Autodesk Inventor part; units mm, degrees
ref_plane "YZ Plane" through (0, 0, 0) normal (1, 0, 0) x (0, 1, 0)
ref_plane "XZ Plane" through (0, 0, 0) normal (0, 1, 0) x (-1, 0, 0)
ref_plane "XY Plane" through (0, 0, 0) normal (0, 0, 1) x (1, 0, 0)
sketch "Sketch1" plane through (0, 0, 0) normal (0, 1, 0) x (-1, 0, 0)
  line L0 (-81.5, 81.5) -> (81.5, -81.5) construction
  line L1 (-81.5, -81.5) -> (81.5, 81.5) construction
  line L2 (-66.3, 66.3) -> (66.3, -66.3) construction
  line L3 (-66.3, -66.3) -> (66.3, 66.3) construction
  line L4 (-81.9, 81.9) -> (-81.9, -81.9)
  line L5 (-81.9, -81.9) -> (81.9, -81.9)
  line L6 (81.9, -81.9) -> (81.9, 81.9)
  line L7 (81.9, 81.9) -> (-81.9, 81.9)
  line L8 (-66.1, 66.1) -> (-66.1, -66.1)
  line L9 (-66.1, -66.1) -> (66.1, -66.1)
  line L10 (66.1, -66.1) -> (66.1, 66.1)
  line L11 (66.1, 66.1) -> (-66.1, 66.1)
  line L12 (-66.1, 66.1) -> (66.1, -66.1) construction
  line L13 (-66.1, -66.1) -> (66.1, 66.1) construction
  line L14 (66.1, 51.9579) -> (17.2261, 3.084)
  line L15 (51.9579, 66.1) -> (3.084, 17.2261)
  line L16 (66.1, -51.9579) -> (14.1421, 0) construction
  line L17 (50.106, -64.2481) -> (3.084, -17.2261)
  arc A0 (-17.2261, -3.084) -> (-3.084, -17.2261) centre (0, 0) ccw
  arc A1 (-17.2261, 3.084) -> (-17.2261, -3.084) centre (0, 0) ccw
  line L18 (-14.1421, 0) -> (-17.2261, -3.084) construction
  line L19 (-3.084, 17.2261) -> (-51.9579, 66.1)
  line L20 (3.084, 17.2261) -> (0, 14.1421) construction
  line L21 (0, 14.1421) -> (-14.1421, 0) construction
  line L22 (14.1421, 0) -> (-3.084, 17.2261) construction
  arc A2 (17.2261, 3.084) -> (-17.2261, 3.084) centre (0, 0) ccw
  arc A3 (17.2261, -3.084) -> (17.2261, 3.084) centre (0, 0) ccw
  arc A4 (-3.084, -17.2261) -> (17.2261, -3.084) centre (0, 0) ccw
  line L23 (3.084, -17.2261) -> (0, -14.1421) construction
  line L24 (0, -14.1421) -> (-14.1421, 0) construction
  line L25 (17.2261, 3.084) -> (-3.084, -17.2261) construction
  line L26 (-3.084, -17.2261) -> (-51.9579, -66.1)
  line L27 (-17.2261, -3.084) -> (-66.1, -51.9579)
  line L28 (-17.2261, 3.084) -> (-64.2481, 50.106)
  line L29 (-14.1421, 0) -> (-17.2261, 3.084) construction
  line L30 (17.2261, -3.084) -> (66.1, -51.9579)
  line L31 (50.106, -64.2481) -> (51.9579, -66.1)
  line L32 (-64.2481, 50.106) -> (-66.1, 51.9579)
  line L33 (46.2, 46.2) -> (-46.2, 46.2) construction
  line L34 (-46.2, 46.2) -> (-46.2, -46.2) construction
  line L35 (-46.2, -46.2) -> (46.2, -46.2) construction
  line L36 (46.2, -46.2) -> (46.2, 46.2) construction
  line L37 (46.2, 46.2) -> (-46.2, -46.2) construction
  line L38 (-46.2, 46.2) -> (46.2, -46.2) construction
  circle A5 centre (46.2, -46.2) radius 1
  circle A6 centre (-46.2, -46.2) radius 1
  circle A7 centre (-46.2, 46.2) radius 1
  circle A8 centre (46.2, 46.2) radius 1
  line L39 (51.9579, 66.1) -> (66.1, 51.9579)
  line L40 (66.1, -51.9579) -> (51.9579, -66.1)
  line L41 (-51.9579, -66.1) -> (-66.1, -51.9579)
  line L42 (-66.1, 51.9579) -> (-51.9579, 66.1)
  line L43 (-74, 74) -> (-74, -74)
  line L44 (-74, -74) -> (74, -74)
  line L45 (74, -74) -> (74, 74)
  line L46 (74, 74) -> (-74, 74)
  line L47 (-74, 74) -> (74, -74) construction
  line L48 (-74, -74) -> (74, 74) construction
  dimension "d0" = 163
  dimension "d1" = 163
  dimension "d2" = 132.6
  dimension "d3" = 132.6
  dimension "d5" = 163.8
  dimension "d6" = 163.8
  dimension "d7" = 132.2
  dimension "d8" = 132.2
  dimension "d9" = 20
  dimension "d10" = 20
  dimension "d11" = 35
  dimension "d12" = 92.4
  dimension "d13" = 92.4
  dimension "d14" = 2
  dimension "d15" = 2
  dimension "d16" = 2
  dimension "d17" = 2
  dimension "d28" = 148
  dimension "d29" = 148
extrude "Extrusion1" add sketch "Sketch1" along normal blind 5 contours L7 L6 L5 L4 | L46 L45 L44 L43
extrude "Extrusion2" add sketch "Sketch1" along normal blind 5 contours L11 L42 L8 | L41 L9 L8 | L11 L10 L39 | L40 L10 L9
extrude "Extrusion4" cut sketch "Sketch1" against normal blind 10 contours L11 L42 L8 | L42 L19 A2 L28 L32 | L41 L9 L8 | L27 A0 L26 L41 | L39 L14 A2 L15 | L11 L10 L39 | A2 A3 A4 A0 A1 | L40 L10 L9 | L31 L17 A4 L30 L40 | A7
extrude "Extrusion5" add sketch "Sketch1" against normal blind 8 contours L11 L42 L8 | L42 L19 A2 L28 L32 | L41 L9 L8 | L27 A0 L26 L41 | L39 L14 A2 L15 | L11 L10 L39 | A2 A3 A4 A0 A1 | L40 L10 L9 | L31 L17 A4 L30 L40
extrude "Extrusion6" cut sketch "Sketch1" along normal blind 8 contours L7 L6 L5 L4
properties part number "Lifting Motor Platform"
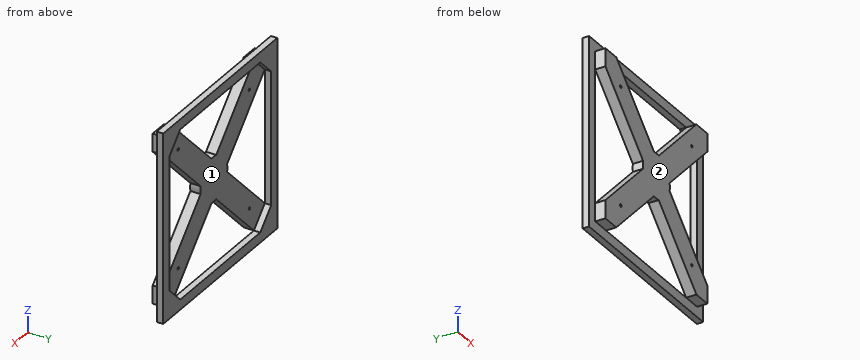
Design review of the part built by this model. Coordinates are the model's own, in mm. Face numbers are marked on the shaded views. Coordinates: 2 decimals unless noted, no trailing zeros. Order: outer loops, then holes, each group sorted by start corner. A loop starts at its lowest first (then second) coordinate and runs counter-clockwise, first axis right, second up. Notation, with made-up numbers: M -9,86.25 L -1,86.25 A22 cw -1,98.25 Z; hole C -27.5,29 d8. An arc over 180 degrees is marked long. Answer as a JSON object with one key per item and string values. Group by question number.
1) Add section B-B, the plane z = -59.5. Write out the cut boundary in (x, y).
2) Mouldability with a two-part tool opening along Z and no side actions: class the marked faces 1 and 2 as pulls with the +Z half, pulls with the -Z half, needs draft (parallel to the pull), parting line crosses it, or undercut.
3) Add section A-A, the plane y = -5.5. Write out the cut boundary in (x, z), then the cut area to 3 significant figures.
4) Add section D-D, the plane x = -6. Write out the cut boundary in (y, z), then the cut area to 3 significant figures.
5) For pin 1 (2 mm diameter, centred on y = -1.5, z = 19, fed in from -X); pin 2 (2 mm diameter, centred on y = -5, z = -37.5, fed in from +X); pin 3 (2.5 mm diameter, centred on y = -2.5, z = -57, fed in from -X), all flat-tipped, find the tip position at first contact; note any pin that passes through.
6) Wall thickness on L1, parallel to X at y = 1.25, z = 37; L2, parallel to Z at x = -46.2, y = -2.75; L3, parallel to Y at x = -41.5, z = -37: over which ranges is each line inside the solid? List them lowest first.
7) Add section C-C, the plane y = 2. Write out the cut boundary in (x, z), then the cut area to 3 significant figures.
Computed values:
{
 "1": {"outline": "M -74,0 L -66.1,0 L -66.1,-8 L -45.36,-8 L -45.36,0 L -58.56,0 L -58.56,5 L -74,5 Z; M 45.36,-8 L 66.1,-8 L 66.1,0 L 74,0 L 74,5 L 58.56,5 L 58.56,0 L 45.36,0 Z"},
 "2": {"face 1": "undercut", "face 2": "needs draft"},
 "3": {"outline": "M -66.1,-66.1 L -51.96,-66.1 L -3.08,-17.23 A17.5 ccw 3.08,-17.23 L 51.96,-66.1 L 66.1,-66.1 L 66.1,-51.96 L 17.23,-3.08 A17.5 ccw 17.23,3.08 L 66.1,51.96 L 66.1,66.1 L 51.96,66.1 L 3.08,17.23 A17.5 ccw -3.08,17.23 L -51.96,66.1 L -66.1,66.1 L -66.1,51.96 L -17.23,3.08 A17.5 ccw -17.23,-3.08 L -66.1,-51.96 Z; hole C -46.2,-46.2 d2; hole C -46.2,46.2 d2; hole C 46.2,-46.2 d2; hole C 46.2,46.2 d2", "area": "6,710 mm^2"},
 "4": {"outline": "M -8,-20.14 L 0,-20.14 L 0,20.14 L -8,20.14 Z; M 0,-74 L 5,-74 L 5,-66.1 L 0,-66.1 Z; M 0,66.1 L 5,66.1 L 5,74 L 0,74 Z", "area": "401 mm^2"},
 "5": {"pin 1": "stops at x = -34.14", "pin 2": "stops at x = 52.64", "pin 3": "stops at x = -66.1"},
 "6": {"L1": "x = -74 to -66.1, 66.1 to 74", "L2": "z = -60.34 to -47.2, -45.2 to -32.06, 32.06 to 45.2, 47.2 to 60.34", "L3": "y = -8 to 0"},
 "7": {"outline": "M -74,-74 L 74,-74 L 74,74 L -74,74 Z; hole M -66.1,-51.96 L -51.96,-66.1 L 51.96,-66.1 L 66.1,-51.96 L 66.1,51.96 L 51.96,66.1 L -51.96,66.1 L -66.1,51.96 Z", "area": "4,830 mm^2"}
}
